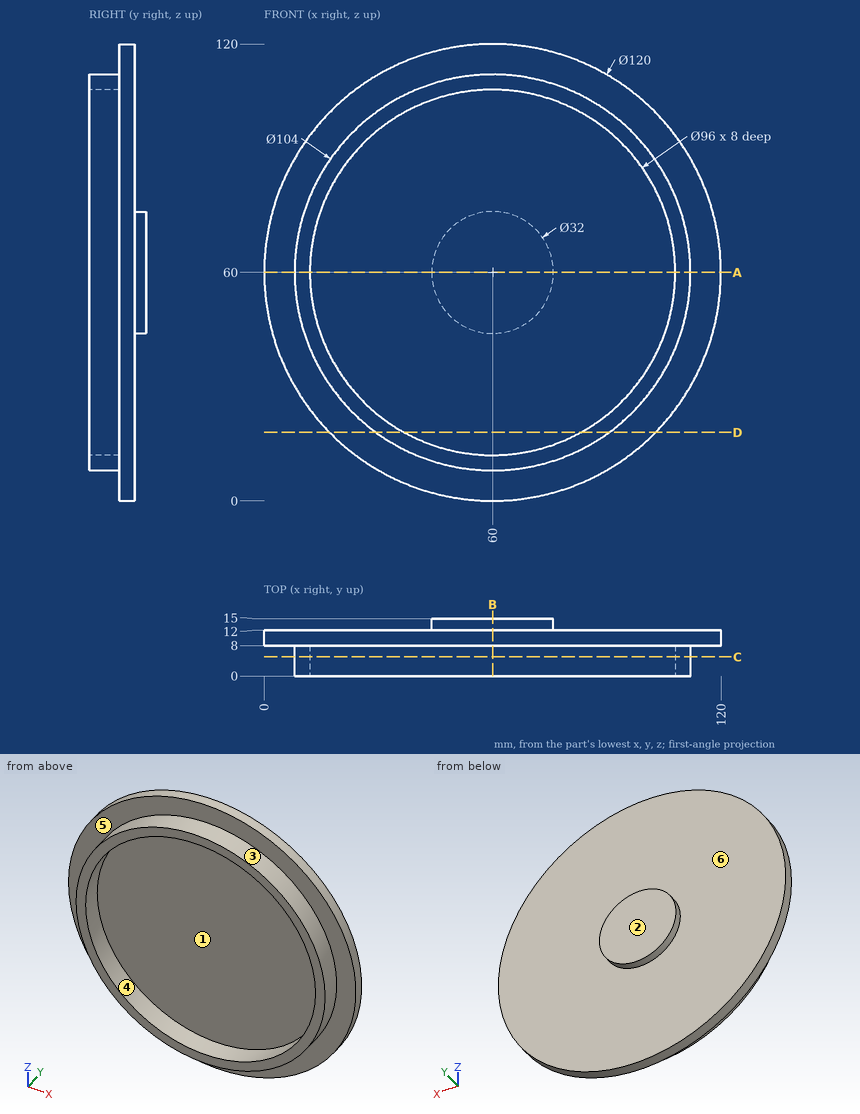
Check sheet for the drawn part. Datum: minimum x, y, z corner. Units: mm. A direction names the side the tool comes from. Give positions to 0.01 mm unless a question says otherwise; leave off trailing zeros. Write each loop counter-clockwise with the first axis right and the second up, starting at its lowest first coordinate (ties: lowest second). Pieces come first, ordered by that corner, then holes. Notation, with made-up numbers: (25, 6) -> (49, 6) arc R21 cw to (49, 12) -> close; hole circle Ø6 at (49, 55). An arc over 180 degrees is marked (long way). Use one line per item in the form item = value. Start each with the question number.
1. Section check A-A (z = 60). Record the cut outline in (x, y), and give its area (3 significant figures).
2. Access from +Z, -Z, +X, -X, +Y, -Y to the whole of each face (thin tool, end or side, straight path). Record for the marked faces 5 and 6.
3. Mould release check, pull along X, two halves, no side actions. Record for the marked faces 1, 2, 3 and 4: pulls with the +X half, pulls with the -X half, needs draft (parallel to the pull), parting line crosses it, or undercut.
4. Section check B-B (x = 60). Record the cut outline in (y, z).
5. Thickness scan on line 1 along Z through (x, y) = (60, 3); line 2 along Y through (x, z) = (98.5, 92); line 3 along Y through (x, z) = (65, 103). Record the ranges inside material, lowest first. Write a range as from..to.
6. Section check C-C (y = 5). Record the cut outline in (x, z), and give its area (3 significant figures).
7. Go/stop test with flat-tipped pins: P1, Ø5, axis at y = 11, z = 44.5, coming from the -X side; P2, Ø5, axis at x = 37, z = 28, coming from the +Y side; P3, Ø6, axis at x = 97, y = 6, coming from the +Z side. Record where each tip stops, or that it passes through.
8. Section check D-D (z = 18). Record the cut outline in (x, y).
Conclusion:
q1.outline = (0, 8) -> (8, 8) -> (8, 0) -> (12, 0) -> (12, 8) -> (108, 8) -> (108, 0) -> (112, 0) -> (112, 8) -> (120, 8) -> (120, 12) -> (76, 12) -> (76, 15) -> (44, 15) -> (44, 12) -> (0, 12) -> close
q1.area = 640 mm²
q2.face_5 = -Y
q2.face_6 = +Y
q3.face_1 = undercut
q3.face_2 = needs draft
q3.face_3 = parting line crosses it
q3.face_4 = undercut
q4.outline = (0, 8) -> (8, 8) -> (8, 0) -> (12, 0) -> (12, 44) -> (15, 44) -> (15, 76) -> (12, 76) -> (12, 120) -> (8, 120) -> (8, 112) -> (0, 112) -> (0, 108) -> (8, 108) -> (8, 12) -> (0, 12) -> close
q5.line_1 = 8..12, 108..112
q5.line_2 = 0..12
q5.line_3 = 8..12
q6.outline = circle Ø104 at (60, 60); hole circle Ø96 at (60, 60)
q6.area = 1,260 mm²
q7.P1 = 1.43
q7.P2 = 12
q7.P3 = 108.9
q8.outline = (17.15, 8) -> (29.34, 8) -> (29.34, 0) -> (36.76, 0) -> (36.76, 8) -> (83.24, 8) -> (83.24, 0) -> (90.66, 0) -> (90.66, 8) -> (102.85, 8) -> (102.85, 12) -> (17.15, 12) -> close
